from build123d import *

# Parameters (mm, degrees)
BOSS_EXTRUDE2_DEPTH      = 2
BOSS_EXTRUDE4_DEPTH      = 4
CUT_EXTRUDE6_DEPTH       = 22.75
SKETCH4_R                = 5.75
CUT_EXTRUDE7_DEPTH       = 2
CUT_EXTRUDE8_DEPTH       = 4
BOSS_EXTRUDE5_DEPTH      = 27
BOSS_EXTRUDE6_DEPTH      = 2
BOSS_EXTRUDE7_DEPTH      = 2
BOSS_EXTRUDE8_DEPTH      = 25
CUT_EXTRUDE10_DEPTH      = 26
SKETCH14_R               = 3.25
CUT_EXTRUDE11_DEPTH      = 1
CUT_EXTRUDE11_DEPTH_BACK = 43.5
CUT_EXTRUDE12_DEPTH      = 1


with BuildPart() as part:
    # Sketch1 → Boss-Extrude2 (new body)
    with BuildSketch(Plane(origin=(0, 0, 0), x_dir=(1, 0, 0), z_dir=(0, 1, 0))):
        with BuildLine():
            Line((-15, 39.764934301), (-15, 20.264934301))
            ThreePointArc((-15, 20.264934301), (0, 25.212448557), (15, 20.264934301))
            Line((15, 20.264934301), (15, 39.764934301))
            ThreePointArc((15, 39.764934301), (0, 42.5), (-15, 39.764934301))
        make_face()
    extrude(amount=BOSS_EXTRUDE2_DEPTH)

    # Sketch2 → Boss-Extrude4 (add)
    with BuildSketch(Plane.XZ):
        with BuildLine():
            Line((6.75, -24.292078179), (6.75, -41.960546946))
            ThreePointArc((6.75, -41.960546946), (0, -42.5), (-6.75, -41.960546946))
            Line((-6.75, -41.960546946), (-6.75, -24.292078179))
            ThreePointArc((-6.75, -24.292078179), (0, -25.212448557), (6.75, -24.292078179))
        make_face()
    extrude(amount=BOSS_EXTRUDE4_DEPTH)

    # Sketch3 → Cut-Extrude6 (cut, through all)
    with BuildSketch(Plane(origin=(6.75, 0, 0), x_dir=(0, 0, -1), z_dir=(1, 0, 0))):
        Polygon((41.960546946, -4), (24.292078179, -2), (24.292078179, -4), align=None)
    extrude(amount=-CUT_EXTRUDE6_DEPTH, mode=Mode.SUBTRACT)

    # Sketch4 → Cut-Extrude7 (cut)
    with BuildSketch(Plane(origin=(0, 0.740280631, -0.083796807), x_dir=(-1, 0, 0), z_dir=(0, -0.993654251, 0.112477687))):
        with Locations((0, 33.039130231)):
            Circle(SKETCH4_R)
    extrude(amount=-CUT_EXTRUDE7_DEPTH, mode=Mode.SUBTRACT)

    # Sketch5 → Cut-Extrude8 (cut)
    with BuildSketch(Plane(origin=(0, 2, 0), x_dir=(1, 0, 0), z_dir=(0, 1, 0))):
        with BuildLine():
            ThreePointArc((-5.75, 40.089743077), (0, 40.5), (5.75, 40.089743077))
            Line((5.75, 40.089743077), (5.75, 26.598023544))
            ThreePointArc((5.75, 26.598023544), (0, 27.212448557), (-5.75, 26.598023544))
            Line((-5.75, 26.598023544), (-5.75, 40.089743077))
        make_face()
    extrude(amount=-CUT_EXTRUDE8_DEPTH, mode=Mode.SUBTRACT)

    # Sketch7 → Boss-Extrude5 (add)
    with BuildSketch(Plane(origin=(0, 2, 0), x_dir=(1, 0, 0), z_dir=(0, 1, 0))):
        with BuildLine():
            Line((-15, 37.619808612), (-15, 39.764934301))
            ThreePointArc((-15, 39.764934301), (0, 42.5), (15, 39.764934301))
            Line((15, 39.764934301), (15, 37.619808612))
            ThreePointArc((15, 37.619808612), (0, 40.5), (-15, 37.619808612))
        make_face()
    extrude(amount=BOSS_EXTRUDE5_DEPTH)

    # Sketch8 → Boss-Extrude6 (add)
    with BuildSketch(Plane(origin=(0, 2, 0), x_dir=(1, 0, 0), z_dir=(0, 1, 0))):
        with BuildLine():
            Line((-15, 22.7050073), (-15, 20.264934301))
            ThreePointArc((-15, 20.264934301), (0, 25.212448557), (15, 20.264934301))
            Line((15, 20.264934301), (15, 22.7050073))
            ThreePointArc((15, 22.7050073), (0, 27.212448557), (-15, 22.7050073))
        make_face()
    extrude(amount=BOSS_EXTRUDE6_DEPTH)

    # Sketch9 → Boss-Extrude7 (add)
    with BuildSketch(Plane(origin=(0, 2, 0), x_dir=(1, 0, 0), z_dir=(0, 1, 0))):
        with BuildLine():
            Line((-15, 37.619808612), (-15, 22.7050073))
            ThreePointArc((-15, 22.7050073), (-14.012881704, 23.32716234), (-13, 23.906429187))
            Line((-13, 23.906429187), (-13, 38.356876828))
            ThreePointArc((-13, 38.356876828), (-14.004849781, 38.001502373), (-15, 37.619808612))
        make_face()
    boss_extrude7 = extrude(amount=BOSS_EXTRUDE7_DEPTH)

    # Mirror1: Boss-Extrude7 across plane
    add(boss_extrude7.mirror(Plane(origin=(0, 0, 0), x_dir=(0, 0, 1), z_dir=(1, 0, 0))))

    # Sketch12 → Boss-Extrude8 (add)
    with BuildSketch(Plane(origin=(0, 4, 0), x_dir=(1, 0, 0), z_dir=(0, 1, 0))):
        with BuildLine():
            ThreePointArc((-13, 38.356876828), (-14.004849781, 38.001502373), (-15, 37.619808612))
            Line((-15, 37.619808612), (-15, 35.619808612))
            Line((-15, 35.619808612), (-13, 35.619808612))
            Line((-13, 35.619808612), (-13, 38.356876828))
        make_face()
        with BuildLine():
            Line((15, 35.619808612), (15, 37.619808612))
            ThreePointArc((15, 37.619808612), (14.004849781, 38.001502373), (13, 38.356876828))
            Line((13, 38.356876828), (13, 35.619808612))
            Line((13, 35.619808612), (15, 35.619808612))
        make_face()
    extrude(amount=BOSS_EXTRUDE8_DEPTH)

    # Sketch13 → Cut-Extrude10 (cut)
    with BuildSketch(Plane(origin=(0, 29, 0), x_dir=(1, 0, 0), z_dir=(0, 1, 0))):
        with BuildLine():
            Line((-14.25, 21.702217285), (-14.25, 36.513007281))
            Line((-14.25, 36.513007281), (-15, 36.513007281))
            Line((-15, 36.513007281), (-15, 20.264934301))
            ThreePointArc((-15, 20.264934301), (0, 25.212448557), (15, 20.264934301))
            Line((15, 20.264934301), (15, 36.513007281))
            Line((15, 36.513007281), (14.25, 36.513007281))
            Line((14.25, 36.513007281), (14.25, 21.702217285))
            ThreePointArc((14.25, 21.702217285), (0, 25.962448557), (-14.25, 21.702217285))
        make_face()
    extrude(amount=-CUT_EXTRUDE10_DEPTH, mode=Mode.SUBTRACT)

    # Sketch14 → Cut-Extrude11 (cut, two sides)
    with BuildSketch(Plane.XY) as cut_extrude11_sk:
        with Locations((0, 29)):
            Circle(SKETCH14_R)
    extrude(amount=CUT_EXTRUDE11_DEPTH, mode=Mode.SUBTRACT)
    extrude(cut_extrude11_sk.sketch, amount=-CUT_EXTRUDE11_DEPTH_BACK, mode=Mode.SUBTRACT)

    # Sketch15 → Cut-Extrude12 (cut)
    with BuildSketch(Plane(origin=(0, 29, 0), x_dir=(1, 0, 0), z_dir=(0, 1, 0))):
        with BuildLine():
            Line((-15, 36.513007281), (-15, 39.764934301))
            ThreePointArc((-15, 39.764934301), (0, 42.5), (15, 39.764934301))
            Line((15, 39.764934301), (15, 36.513007281))
            Line((15, 36.513007281), (14.25, 36.513007281))
            Line((14.25, 36.513007281), (14.25, 39.242833741))
            ThreePointArc((14.25, 39.242833741), (0, 41.75), (-14.25, 39.242833741))
            Line((-14.25, 39.242833741), (-14.25, 36.513007281))
            Line((-14.25, 36.513007281), (-15, 36.513007281))
        make_face()
    extrude(amount=-CUT_EXTRUDE12_DEPTH, mode=Mode.SUBTRACT)


solid = part.part
Geometry check sheet. Reference: the model listing, model coordinates, mm. A direction names the side the tool comes from. Round coordinates to 2 decimals unless told otherwise and drop trailing zeros. Order: outer loops, then holes, each group sorted by start corner. A loop starts at its lowest first (then second) coordinate and runs counter-clockwise, first axis right, second up. Notation, with made-up numbers: (80, 55.5) - (106, 55.5) arc R28 cw to (106, 85.5) - close; hole circle Ø4 at (70.25, 54.5). An arc over 180 degrees is marked (long way). One line per question, with ' | ' between items. Start each with the question number.
(1) Access from +Z, -Z, +X, -X, +Y, -Y to the whole of each face (thin tool, end or side, straight path). Record for faces 4 (the flat face through (-10, 28, -41)), 5 (the flat face through (5.75, 0, -33)), 6 (the flat face through (-6.75, -2, -33)), 7 (the flat face through (0, 4, -27)).
(2) Sectioned sample at B-B on y = 0.5. Record the cut outline in (x, z).
(3) Depth check by flat-ended pin: pin 1 Ø2 at (x, y) = (-7.5, 1.5) entering from -Z; pin 2 Ø1.5 at (x, y) = (-4.5, 18.5) entering from +Z; pin 3 Ø0.8 at (x, y) = (14.5, 19.5) entering from +Z. Enter the tip coordinate at first touch or a pass-through.
(4) Thickness scan on L1, parallel to X at y = -1, z = -36.25; L2, parallel to X at y = 13.5, z = -37.5; L3, parallel to Y at x = 7.5, z = -30.75. Record the ranges inside material, lowest first. Write a range as [from, to].
(5) Sectioned sample at D-D on y = 5. Record the cut outline in (x, z).
(6) Release check for a two-part mould opening along Z. For faces 1 (the flat face through (-11, 0, -31)), 2 (the flat face through (-9, 2, -32)), 3 (the flat face through (-14, 16, -35.62)) record: released by +Z, released by -Z, zero draft, split by the parting line, or undercut.
(7) Sectioned sample at C-C on z = -22.5. Record the cut outline in (x, y), and give its area (3 significant figures).
Conclusion:
1) face 4: -Z, -X, +Y | face 5: +Y | face 6: +Z, -Z, -X, -Y | face 7: +Z, +X, -X, +Y
2) outline: (-15, -39.76) arc R42.5 ccw to (15, -39.76) - (15, -20.26) arc R25.21 cw to (-15, -20.26) - close; hole (-5.75, -40.09) arc R40.5 ccw to (5.75, -40.09) - (5.75, -26.6) arc R27.21 cw to (-5.75, -26.6) - close
3) pin 1: stops at z = -42 | pin 2: stops at z = -40.16 | pin 3: stops at z = -35.62
4) L1: x = [-6.75, -5.75], [5.75, 6.75] | L2: x = [-15, -13], [13, 15] | L3: y = [0, 2]
5) outline: (-15, -39.76) arc R42.5 ccw to (15, -39.76) - (15, -36.51) - (14.25, -36.51) - (14.25, -35.62) - (13, -35.62) - (13, -38.36) arc R40.5 cw to (-13, -38.36) - (-13, -35.62) - (-14.25, -35.62) - (-14.25, -36.51) - (-15, -36.51) - close
6) face 1: zero draft | face 2: undercut | face 3: released by +Z
7) outline: (-15, 0) - (-11.38, 0) - (-11.38, 3) - (-12.95, 3) - (-12.95, 4) - (-14.25, 4) - (-14.25, 3) - (-15, 3) - close; (11.38, 0) - (15, 0) - (15, 3) - (14.25, 3) - (14.25, 4) - (12.95, 4) - (12.95, 3) - (11.38, 3) - close | area: 24.3 mm2
